Geometry check sheet. Reference: the model listing, model coordinates, mm. A direction names the side the tool comes from. Round coordinates to 2 decimals unless told otherwise and drop trailing zeros. Loops run counter-clockwise (first coordinate to the right, second up) from the corner with the lowest first, then second, coordinate; pieces in that order, holes last. Notation, with made-up numbers: (65.5, 7) -> (115.5, 7) arc R21 cw to (115.5, 14) -> close; hole circle Ø8 at (60, 47.25). An arc over 180 degrees is marked (long way). Use a Markdown table: item, result. Add a question column.
Q1. Sectioned sample at D-D, the plane y = 32.5. Enter the section's corners in (x, z) (3 decimals), then the cut area to 3 significant figures.
Q2. Sectioned sample at B-B, the plane z = 0. Enter the section's corners in (x, y), then the cut area to 3 significant figures.
Q3. Set-up check for faces 1 (the face through (3, -22.035, -15)), 2 (the face through (-21.715, 143.194, 0.128)), 3 (the face through (17.894, -24.14, 14.548)), 4 (the face through (-7.3, 72.3, -4.41)), 5 (the face through (2.855, 18.554, 4.41)): record each of +Z, -Z, +X, -X, +Y, -Y from which the full face is reachable in a straight line by a thin tool's end or side.
Q4. Sectioned sample at C-C, the plane y = 0. Enter the section's corners in (x, z) (3 decimals), then the cut area to 3 significant figures.
Q5. Material ranges on L1, parallel to X at y = 0, z = -3; L2, parallel to Y at x = 0, z = -3.75; L3, parallel to Y at x = 2, z = -10, recorded low to high.
Q6. Gauge pin test, flat ends, axial feed: P1, Ø10, axis at x = 9.5, y = -31.5, coming from the -Z side (3 decimals); P2, Ø4, axis at x = 4.5, y = 126.5, coming from the +Z side; P3, Ø16.5, axis at x = 0, y = 0, coming from the +Z side (3 decimals). Record the tip position at first contact, or that the pin passes through.
Q7. Release check for a two-part mould opening along X. For faces 6 (the face through (-47.57, 160.554, -0.128)), 7 (the face through (-12.114, -24.14, -14.702)), 8 (the face through (-48, 180, 25.4)) record: released by +X, released by -X, zero draft, split by the parting line, or undercut.
Q8. Sectioned sample at A-A, the plane y = -40.52. Enter the section's corners in (x, z) (3 decimals), then the cut area to 3 significant figures.
```python
from build123d import *
from build123d.topology import SkipClean

# Parameters (mm, degrees)
SKETCH2_R               = 6.3999999999999995
SKETCH2_R_2             = 12.920000000000002
BOSS_EXTRUDE1_DEPTH     = 20.125
BOSS_EXTRUDE2_DEPTH     = 25.4
CUT_EXTRUDE1_DEPTH      = 17.625
FILLET2_R               = 9.525
FILLET1_R               = 6.35
FILLET2_OF_MIRROR1_R    = 9.525
FILLET1_OF_MIRROR1_R    = 6.35
CUT_EXTRUDE3_REACH      = 230.532
CUT_EXTRUDE3_END_RADIUS = 87.85596312436087
CUT_EXTRUDE4_DEPTH      = 34
FILLET3_R               = 6.35
CUT_EXTRUDE6_DEPTH      = 11
FILLET4_R               = 7


with BuildPart() as part:
    # Sketch2 → Boss-Extrude1 (new, symmetric)
    with BuildSketch(Plane.XY):
        with BuildLine():
            Line((-14.110000000000005, 117.05420999809479), (-14.110000000000003, 39.41472795492869))
            Line((-14.110000000000003, 39.41472795492869), (-14.109999999999992, -58.249999999999986))
            Line((-14.109999999999992, -58.24999999999999), (19.890000000000008, -58.24999999999999))
            Line((19.89000000000001, -58.24999999999999), (19.89000000000001, 39.414727954928686))
            Line((19.89000000000001, 39.41472795492869), (19.89000000000001, 116.74999999999999))
            ThreePointArc((19.890000000000022, 116.74999999999999), (2.3016026864285166, 165.96310053609741), (-42.49516565662927, 192.88020532941604))
            ThreePointArc((-42.49516565662924, 192.88020532941601), (-47.59126491681772, 178.8312081202326), (-50.2324931256602, 164.12173961174625))
            ThreePointArc((-50.23249312566025, 164.12173961174625), (-24.181503081041093, 146.71979128999487), (-14.110000000000007, 117.05420999809479))
        make_face()
        Circle(SKETCH2_R, mode=Mode.SUBTRACT)
        with Locations((2.160000000000005, -40.52)):
            Circle(SKETCH2_R_2, mode=Mode.SUBTRACT)
    extrude(amount=BOSS_EXTRUDE1_DEPTH, both=True)

    # Sketch2<3> → Boss-Extrude2 (add, symmetric)
    with BuildSketch(Plane.XY):
        with BuildLine():
            Line((-55.11000000000002, 146.4), (-50.13682514315135, 146.9172348047148))
            ThreePointArc((-50.13682514315135, 146.9172348047148), (-47.01837422138325, 180.86294224819565), (-31.213761902356293, 211.06641919101017))
            Line((-31.213761902356293, 211.06641919101017), (-35.11000000000003, 214.2))
            ThreePointArc((-35.11000000000003, 214.2), (-51.814073878435075, 182.27760291399264), (-55.11000000000002, 146.4))
        make_face()
    extrude(amount=BOSS_EXTRUDE2_DEPTH, both=True)

    # Sketch3 → Cut-Extrude1 (cut)
    with BuildSketch(Plane.XY.offset(20.125)):
        with BuildLine():
            Line((-9.109999999999992, 16.74326446705436), (-9.110000000000003, 117.05420999809479))
            ThreePointArc((-9.110000000000003, 117.05420999809479), (-20.430838112311193, 150.0432736077851), (-49.62239933784868, 169.12972028140788))
            ThreePointArc((-49.62239933784868, 169.12972028140788), (-47.60047450986274, 178.79694990145757), (-44.50629280792827, 188.17615819065796))
            ThreePointArc((-44.50629280792827, 188.17615819065796), (-1.899187077854016, 163.1978623652425), (14.890000000000011, 116.74999999999999))
            Line((14.890000000000011, 116.74999999999999), (14.890000000000011, 16.74326446705436))
            Line((14.890000000000011, 16.74326446705436), (-9.109999999999992, 16.74326446705436))
        make_face()
    cut_extrude1 = extrude(amount=-CUT_EXTRUDE1_DEPTH, mode=Mode.SUBTRACT)

    # Fillet2
    fillet2_edges = [part.edges().sort_by_distance(p)[0] for p in [
        (14.890000000000011, 16.74326446705436, 11.3125),
        (-9.109999999999992, 16.74326446705436, 11.3125),
    ]]
    fillet(fillet2_edges, radius=FILLET2_R)

    # Fillet1
    fillet1_edges = [part.edges().sort_by_distance(p)[0] for p in [
        (-20.430838112311193, 150.0432736077851, 2.5),
        (-47.600474509862764, 178.79694990145757, 2.5),
        (-49.62239933784869, 169.12972028140788, 11.3125),
        (-1.8991870778540232, 163.1978623652425, 2.5),
        (-44.506292807928276, 188.17615819065796, 11.3125),
        (-9.109999999999998, 71.66123723257456, 2.5),
        (2.8900000000000112, 16.74326446705436, 2.5),
        (14.890000000000011, 71.50913223352717, 2.5),
        (12.100192090801878, 19.53307237625249, 2.5),
        (-6.32019209080186, 19.53307237625249, 2.5),
    ]]
    fillet(fillet1_edges, radius=FILLET1_R)

    # Mirror1: Cut-Extrude1 across plane
    add(cut_extrude1.mirror(Plane.XY), mode=Mode.SUBTRACT)

    # Fillet2 of Mirror1
    fillet2_of_mirror1_edges = [part.edges().sort_by_distance(p)[0] for p in [
        (14.890000000000011, 16.74326446705436, -11.3125),
        (-9.109999999999992, 16.74326446705436, -11.3125),
    ]]
    fillet(fillet2_of_mirror1_edges, radius=FILLET2_OF_MIRROR1_R)

    # Fillet1 of Mirror1
    fillet1_of_mirror1_edges = [part.edges().sort_by_distance(p)[0] for p in [
        (-20.430838112311193, 150.0432736077851, -2.5),
        (-47.600474509862764, 178.79694990145757, -2.5),
        (-49.62239933784869, 169.12972028140788, -11.3125),
        (-1.8991870778540232, 163.1978623652425, -2.5),
        (-44.506292807928276, 188.17615819065796, -11.3125),
        (-9.109999999999998, 71.66123723257456, -2.5),
        (2.8900000000000112, 16.74326446705436, -2.5),
        (14.890000000000011, 71.50913223352717, -2.5),
        (12.100192090801878, 19.53307237625249, -2.5),
        (-6.32019209080186, 19.53307237625249, -2.5),
    ]]
    fillet(fillet1_of_mirror1_edges, radius=FILLET1_OF_MIRROR1_R)

    # Cut-Extrude3: up to this cylinder (the profile starts inside it)
    with SkipClean():  # the faces are left unmerged after this step: merging them gives an invalid solid
        cut_extrude3_end = Plane(origin=(37.24778822370744, 156.0056671906468, 17.416667), z_dir=(0, 0, -1)) * Cylinder(CUT_EXTRUDE3_END_RADIUS, 637.7759262487218, mode=Mode.PRIVATE)
        # Sketch5 → Cut-Extrude3 (cut, up to the surface)
        with BuildSketch(Plane(origin=(19.89000000000001, 0, 0), x_dir=(0, 0, -1), z_dir=(1, 0, 0)), mode=Mode.PRIVATE) as cut_extrude3_sk1:
            Polygon((-20.125, 29.25), (-12, 192.88020532941607), (-20.125, 192.88020532941607), align=None)
        cut_extrude3_tool1 = extrude(cut_extrude3_sk1.sketch, amount=-CUT_EXTRUDE3_REACH, mode=Mode.PRIVATE) & cut_extrude3_end
        cut_extrude3 = cut_extrude3_tool1.solids().sort_by_distance((19.89, 138.336804, 17.416667))[0]
        add(cut_extrude3, mode=Mode.SUBTRACT)

    # Sketch5<2> → Cut-Extrude4 (cut)
    with SkipClean():  # the faces are left unmerged after this step: merging them gives an invalid solid
        with BuildSketch(Plane(origin=(19.89000000000001, 0, 0), x_dir=(0, 0, -1), z_dir=(1, 0, 0))):
            Polygon((-20.125, 29.25), (-12, 192.88020532941607), (-20.125, 192.88020532941607), align=None)
        cut_extrude4 = extrude(amount=-CUT_EXTRUDE4_DEPTH, mode=Mode.SUBTRACT)

    # Mirror3: Cut-Extrude3, Cut-Extrude4 across plane
    with SkipClean():  # the faces are left unmerged after this step: merging them gives an invalid solid
        add(cut_extrude3.mirror(Plane.XY), mode=Mode.SUBTRACT)
        add(cut_extrude4.mirror(Plane.XY), mode=Mode.SUBTRACT)

    # Fillet3
    # the kernel refuses this fillet: 6.35 mm, written as the material it adds along each edge
    with BuildSketch(Plane(origin=(-42.49516565662923, 192.88020532941607, 32.81193482848439), x_dir=(0.9695328883801022, -0.24496117722883434, 0), z_dir=(0, 0, -1))) as fillet3_piece_1_section:
        with BuildLine():
            CenterArc((8.024480114111293, -6.3421701367020615), FILLET3_R, 92.84559109505132, 103.22260019601504)
            ThreePointArc((1.922555805727569, -8.099730871002809), (0.8652879633419357, -4.072649651231302), (0, 0))
            ThreePointArc((0, 0), (3.854618709259254, -0.0957393715417783), (7.709237418518542, 1.1e-16))
        make_face()
    fillet3_piece_1 = extrude(amount=65.62386965696876, mode=Mode.PRIVATE)
    fillet3_piece_1 = split(fillet3_piece_1, bisect_by=Plane(origin=(-39.886829020293874, 194.82853980671922, 11.903256140293786), z_dir=(0, -0.04959354560053897, -0.9987694830313786)), keep=Keep.TOP, mode=Mode.PRIVATE)
    fillet3_piece_1 = split(fillet3_piece_1, bisect_by=Plane(origin=(-39.886829020293874, 194.82853980671922, -11.903256140293786), z_dir=(0, -0.04959354560053897, 0.9987694830313786)), keep=Keep.TOP, mode=Mode.PRIVATE)
    add(fillet3_piece_1)
    with BuildSketch(Plane(origin=(-50.2324931256602, 164.12173961174625, -36.817821832007795), x_dir=(0.9366748288378645, -0.3502003212756337, 0), z_dir=(0, 0, 1))) as fillet3_piece_2_section:
        with BuildLine():
            CenterArc((8.74629308675495, -6.320667702743433), FILLET3_R, 84.49076719702147, 116.61848813582492)
            ThreePointArc((2.822407485998928, -8.607604385110362), (1.3001924139031467, -4.340202472151455), (0, 0))
            ThreePointArc((0, 0), (4.6779660766656175, 0.2250766052239502), (9.355932153331263, 2.8e-16))
        make_face()
    fillet3_piece_2 = extrude(amount=73.63564366401559, mode=Mode.PRIVATE)
    fillet3_piece_2 = split(fillet3_piece_2, bisect_by=Plane(origin=(-48.29188317260997, 162.0247617991737, 13.532116140650901), z_dir=(0, -0.04959354560053897, -0.9987694830313786)), keep=Keep.TOP, mode=Mode.PRIVATE)
    fillet3_piece_2 = split(fillet3_piece_2, bisect_by=Plane(origin=(-48.29188317260997, 162.02476179917375, -13.5321161406509), z_dir=(0, -0.04959354560053897, 0.9987694830313786)), keep=Keep.TOP, mode=Mode.PRIVATE)
    add(fillet3_piece_2)

    # Sketch7 → Cut-Extrude6 (cut)
    with SkipClean():  # the faces are left unmerged after this step: merging them gives an invalid solid
        with BuildSketch(Plane.XY.offset(20.125)):
            with BuildLine():
                Line((-22.47666315598992, -22.034869971016057), (33.32085672898189, -22.034869971016057))
                Line((33.32085672898189, -22.034869971016057), (33.32085672898189, 196.87887338600035))
                Line((33.32085672898189, 196.87887338600035), (-31.213761902356293, 211.06641919101017))
                ThreePointArc((-31.213761902356293, 211.06641919101017), (-47.01837422138329, 180.8629422481957), (-50.13682514315135, 146.9172348047148))
                Line((-50.13682514315135, 146.9172348047148), (-22.47666315598992, -22.034869971016057))
            make_face()
        cut_extrude6 = extrude(amount=-CUT_EXTRUDE6_DEPTH, mode=Mode.SUBTRACT)

    # Mirror4: Cut-Extrude6 across plane
    with SkipClean():  # the faces are left unmerged after this step: merging them gives an invalid solid
        add(cut_extrude6.mirror(Plane.XY), mode=Mode.SUBTRACT)

    # Fillet4
    fillet4_edges = [part.edges().sort_by_distance(p)[0] for p in [
        (-14.110000000000001, -22.03486997101606, 14.625),
        (19.89000000000001, -22.034869971016057, 14.625),
        (19.89000000000001, -22.034869971016057, -14.625),
        (-14.110000000000001, -22.03486997101606, -14.625),
    ]]
    fillet(fillet4_edges, radius=FILLET4_R)


solid = part.part
```
Values:
| question | item | result |
|---|---|---|
| 1 | outline | (-14.11, -9.125) -> (-9.11, -9.125) -> (-9.11, -8.85) arc R6.35 cw to (-2.76, -2.5) -> (8.54, -2.5) arc R6.35 cw to (14.89, -8.85) -> (14.89, -9.125) -> (19.89, -9.125) -> (19.89, 9.125) -> (14.89, 9.125) -> (14.89, 8.85) arc R6.35 cw to (8.54, 2.5) -> (-2.76, 2.5) arc R6.35 cw to (-9.11, 8.85) -> (-9.11, 9.125) -> (-14.11, 9.125) -> close |
| 1 | area | 337 mm^2 |
| 2 | outline | (-55.11, 146.4) -> (-50.14, 146.92) arc R87.86 cw to (-50.6, 155.07) arc R6.35 cw to (-41.47, 160.85) arc R48.73 cw to (-14.11, 117.05) -> (-14.11, -58.25) -> (19.89, -58.25) -> (19.89, 116.75) arc R77.64 ccw to (-35.02, 190.99) arc R6.35 cw to (-38.65, 200.26) arc R87.86 cw to (-31.21, 211.07) -> (-35.11, 214.2) arc R92.86 ccw to start; hole circle Ø25.84 at (2.16, -40.52); hole circle Ø12.8 at (0, 0) |
| 2 | area | 8,480 mm^2 |
| 3 | face 1 | -Z, +X, -X, +Y |
| 3 | face 2 | +Z, -Z, -Y |
| 3 | face 3 | +Z, +X, +Y |
| 3 | face 4 | -Z |
| 3 | face 5 | +Z |
| 4 | outline | (-14.11, -9.125) -> (-6.4, -9.125) -> (-6.4, 9.125) -> (-14.11, 9.125) -> close; (6.4, -9.125) -> (19.89, -9.125) -> (19.89, 9.125) -> (6.4, 9.125) -> close |
| 4 | area | 387 mm^2 |
| 5 | L1 | -14.11 to -6.4, 6.4 to 19.89 |
| 5 | L2 | -58.25 to -53.26, -27.78 to -6.4, 6.4 to 19.32, 156.44 to 168.64 |
| 5 | L3 | -58.25 to -53.44, -27.6 to -22.03 |
| 6 | P1 | z = -20.125 |
| 6 | P2 | z = 2.5 |
| 6 | P3 | z = 9.125 |
| 7 | face 6 | undercut |
| 7 | face 7 | released by -X |
| 7 | face 8 | zero draft |
| 8 | outline | (-14.11, -20.125) -> (-10.76, -20.125) -> (-10.76, 20.125) -> (-14.11, 20.125) -> close; (15.08, -20.125) -> (19.89, -20.125) -> (19.89, 20.125) -> (15.08, 20.125) -> close |
| 8 | area | 328 mm^2 |
